```python
from build123d import *

# Parameters (mm, degrees)
BOX032_W                                   = 22
BOX032_H                                   = 24
BOX032_DEPTH                               = 8
CHAMFER004013007011015006009007001004_SIZE = 5
CHAMFER004013007011015006009007001005_SIZE = 0.4


with BuildPart() as part:
    # Box032 → Box032 (new body)
    with BuildSketch(Plane(origin=(11, -12, 16), x_dir=(1, 0, 0), z_dir=(0, 0, 1))):
        with Locations((11, 12)):
            Rectangle(BOX032_W, BOX032_H)
    extrude(amount=BOX032_DEPTH)

    # Chamfer004013007011015006009007001004
    chamfer004013007011015006009007001004_edges = [part.edges().sort_by_distance(p)[0] for p in [
        (33, -12, 20),
        (33, 12, 20),
    ]]
    chamfer(chamfer004013007011015006009007001004_edges, length=CHAMFER004013007011015006009007001004_SIZE)

    # Chamfer004013007011015006009007001005
    chamfer004013007011015006009007001005_edges = [part.edges().sort_by_distance(p)[0] for p in [
        (33, 0, 24),
        (19.5, 12, 24),
        (19.5, -12, 24),
        (30.5, -9.5, 24),
        (30.5, 9.5, 24),
    ]]
    chamfer(chamfer004013007011015006009007001005_edges, length=CHAMFER004013007011015006009007001005_SIZE)


solid = part.part
```
Design review of the part built by this model. Coordinates are the model's own, in mm. Coordinates: 2 decimals unless noted, no trailing zeros. Order: outer loops, then holes, each group sorted by start corner. A loop starts at its lowest first (then second) coordinate and runs counter-clockwise, first axis right, second up. Notation, with made-up numbers: (45, 82) -> (102, 82) arc R7 ccw to (102, 94) -> close; hole circle Ø3 at (-1, 79). An arc over 180 degrees is marked (long way). One line per item, written item: value. Start each with the question number.
Q1. Take a section at B-B, the plane y = 10.5. State the section outline as (x, z) points.
Q2. Take a section at A-A, the plane z = 22.25. State the section outline as (x, y) points, then the cut area to 3 significant figures.
Q3. Take a section at C-C, the plane x = 31.75. State the section outline as (y, z) points.
Q4. For probe 1 along Y at (x, z) = (28.75, 19); probe 2 along Y at (x, z) = (29.25, 18.5); probe 3 along X at (y, z) = (-10.5, 17.25), list the stretches that pass through material, from the lowest coordinate up.
Values follow:
1. outline: (11, 16) -> (29.5, 16) -> (29.5, 23.6) -> (28.93, 24) -> (11, 24) -> close
2. outline: (11, -12) -> (28, -12) -> (33, -7) -> (33, 7) -> (28, 12) -> (11, 12) -> close
2. area: 503 mm2
3. outline: (-8.25, 16) -> (8.25, 16) -> (8.25, 23.6) -> (7.68, 24) -> (-7.68, 24) -> (-8.25, 23.6) -> close
4. probe 1: y = -11.25 to 11.25
4. probe 2: y = -10.75 to 10.75
4. probe 3: x = 11 to 29.5
